```python
from build123d import *

# Parameters (mm, degrees)
SKETCH1_W           = 96.210678118
SKETCH1_H           = 96.210678118
SKETCH1_R           = 10
SKETCH1_R_2         = 3.25
SKETCH1_R_3         = 4.25
BOSS_EXTRUDE1_DEPTH = 60
CUT_EXTRUDE2_DEPTH  = 48
SKETCH2_R           = 5.25
CUT_EXTRUDE3_DEPTH  = 54


with BuildPart() as part:
    # Sketch1 → Boss-Extrude1 (new body)
    with BuildSketch(Plane(origin=(0, 0, 0), x_dir=(1, 0, 0), z_dir=(0, 1, 0))):
        Rectangle(SKETCH1_W, SKETCH1_H)
        with Locations(Location((0, 0, 0), (0, 0, 270))):
            Circle(SKETCH1_R, mode=Mode.SUBTRACT)
        with Locations(Location((0, 15, 0), (0, 0, 270))):
            Circle(SKETCH1_R_2, mode=Mode.SUBTRACT)
        with Locations(Location((35.355339059, 35.355339059, 0), (0, 0, 270))):
            Circle(SKETCH1_R_3, mode=Mode.SUBTRACT)
        with Locations(Location((12.990381057, 7.5, 0), (0, 0, 270))):
            Circle(SKETCH1_R_2, mode=Mode.SUBTRACT)
        with Locations(Location((12.990381057, -7.5, 0), (0, 0, 270))):
            Circle(SKETCH1_R_2, mode=Mode.SUBTRACT)
        with Locations(Location((0, -15, 0), (0, 0, 270))):
            Circle(SKETCH1_R_2, mode=Mode.SUBTRACT)
        with Locations(Location((-12.990381057, -7.5, 0), (0, 0, 270))):
            Circle(SKETCH1_R_2, mode=Mode.SUBTRACT)
        with Locations(Location((-12.990381057, 7.5, 0), (0, 0, 270))):
            Circle(SKETCH1_R_2, mode=Mode.SUBTRACT)
        with Locations(Location((35.355339059, -35.355339059, 0), (0, 0, 270))):
            Circle(SKETCH1_R_3, mode=Mode.SUBTRACT)
        with Locations(Location((-35.355339059, -35.355339059, 0), (0, 0, 270))):
            Circle(SKETCH1_R_3, mode=Mode.SUBTRACT)
        with Locations(Location((-35.355339059, 35.355339059, 0), (0, 0, 270))):
            Circle(SKETCH1_R_3, mode=Mode.SUBTRACT)
    extrude(amount=BOSS_EXTRUDE1_DEPTH)

    # Sketch4 → Cut-Extrude2 (cut)
    with BuildSketch(Plane(origin=(0, 60, 0), x_dir=(1, 0, 0), z_dir=(0, 1, 0))):
        Polygon((-22.605339059, 48.105339059), (22.605339059, 48.105339059), (22.605339059, 22.605339059), (48.105339059, 22.605339059), (48.105339059, -22.605339059), (22.605339059, -22.605339059), (22.605339059, -48.105339059), (-22.605339059, -48.105339059), (-22.605339059, -22.605339059), (-48.105339059, -22.605339059), (-48.105339059, 22.605339059), (-22.605339059, 22.605339059), align=None)
    extrude(amount=-CUT_EXTRUDE2_DEPTH, mode=Mode.SUBTRACT)

    # Sketch2 → Cut-Extrude3 (cut)
    with BuildSketch(Plane(origin=(0, 60, 0), x_dir=(1, 0, 0), z_dir=(0, 1, 0))):
        with Locations((-12.990381057, 7.5)):
            Circle(SKETCH2_R)
        with Locations((0, 15)):
            Circle(SKETCH2_R)
        with Locations((12.990381057, 7.5)):
            Circle(SKETCH2_R)
        with Locations((12.990381057, -7.5)):
            Circle(SKETCH2_R)
        with Locations((0, -15)):
            Circle(SKETCH2_R)
        with Locations((-12.990381057, -7.5)):
            Circle(SKETCH2_R)
    extrude(amount=-CUT_EXTRUDE3_DEPTH, mode=Mode.SUBTRACT)


solid = part.part
```
Source: CAD feature listing. Evaluate the final solid. Frame: model axes, mm. A direction names the side the tool comes from. Give positions to 0.01 mm unless a question says otherwise; leave off trailing zeros. Order: outer loops, then holes, each group sorted by start corner. A loop starts at its lowest first (then second) coordinate and runs counter-clockwise, first axis right, second up.
(1) Section query B-B (y = 25). Return the cut outline in (x, z).
(2) Contact query for flat-ended pins moving along their axis: P1, Ø8.5, axis at x = -12.99, z = -7.5, coming from the -Y side; P2, Ø3, axis at x = -11.5, z = -5, coming from the +Y side; P3, Ø1, axis at x = 7.5, z = -29.5, coming from the +Y side; P4, Ø7, axis at x = 35.36, z = -35.36, coming from the +Y side. Output: stop coordinate, or through.
(3) Access query for faces 1 (the face through (22.605, 36, 35)), 2 (the face through (-36, 36, -22.605)), 3 (the face through (0.212, 9.042, -20.246)). Directions: +Z, -Z, +X, -X, +Y, -Y. A direction counts if a zero-diameter tool reaches every point of the face in a straight line with its end or side. Return the directions, or none.
(4) Section query A-A (z = 0). Return the cut outline in (x, y).
(5) Pull-direction query (X, two-part tool) for faces 4 (the face through (11, 12, -1)), 5 (the face through (-36, 60, -41)), 6 (the face through (48.105, 10, 1)); classes: +X half, -X half, draft (parallel to the pull), parting line (faces both ways), or undercut.
(6) Section query C-C (x = 24.5). Return the cut outline in (y, z).
(7) Material intervals for line 1 along X through (y, z) = (3.5, -35.5); line 2 along Z through (x, y) = (26, 32); line 3 along Z through (x, y) = (3.5, 10), sorted ascending.
(8) Section query D-D (x = 0). Return the cut outline in (y, z), plus the area to 3 significant figures.
Outcome:
1. outline: (-48.11, -48.11) - (-22.61, -48.11) - (-22.61, -22.61) - (-48.11, -22.61) - close; (-48.11, 22.61) - (-22.61, 22.61) - (-22.61, 48.11) - (-48.11, 48.11) - close; (22.61, -48.11) - (48.11, -48.11) - (48.11, -22.61) - (22.61, -22.61) - close; (22.61, 22.61) - (48.11, 22.61) - (48.11, 48.11) - (22.61, 48.11) - close; hole circle Ø8.5 at (-35.36, -35.36); hole circle Ø8.5 at (-35.36, 35.36); hole circle Ø8.5 at (35.36, -35.36); hole circle Ø8.5 at (35.36, 35.36)
2. P1: stops at y = 0
2. P2: stops at y = 6
2. P3: stops at y = 12
2. P4: passes through
3. face 1: +Z, -Z, +Y
3. face 2: +X, -X, +Y
3. face 3: +Y
4. outline: (-48.11, 0) - (-10, 0) - (-10, 12) - (-48.11, 12) - close; (10, 0) - (48.11, 0) - (48.11, 12) - (10, 12) - close
5. face 4: undercut
5. face 5: draft
5. face 6: +X half
6. outline: (0, -48.11) - (60, -48.11) - (60, -22.61) - (12, -22.61) - (12, 22.61) - (60, 22.61) - (60, 48.11) - (0, 48.11) - close
7. line 1: x = -48.11 to -39.6, -31.11 to 31.11, 39.6 to 48.11
7. line 2: z = -48.11 to -22.61, 22.61 to 48.11
7. line 3: z = -48.11 to -18.91, -11.09 to -9.37, 9.37 to 11.09, 18.91 to 48.11
8. outline: (0, -48.11) - (12, -48.11) - (12, -20.25) - (6, -20.25) - (6, -18.25) - (0, -18.25) - close; (0, -11.75) - (6, -11.75) - (6, -10) - (0, -10) - close; (0, 10) - (6, 10) - (6, 11.75) - (0, 11.75) - close; (0, 18.25) - (6, 18.25) - (6, 20.25) - (12, 20.25) - (12, 48.11) - (0, 48.11) - close
8. area: 714 mm2
